Part print with two shaded views. Sizes in mm from the minimum x, y, z corner. Give positions to 0.01 mm unless a question says otherwise; leave off trailing zeros. Order: outer loops, then holes, each group sorted by start corner. A loop starts at its lowest first (then second) coordinate and runs counter-clockwise, first axis right, second up. Notation, with made-up numbers: M 5.5,-13 L 25.5,-13 A29 ccw 25.5,21 Z; hole C 31,-23.75 d7. An arc over 180 degrees is marked long. Return JSON: item names as keys, results as strings. Group by question number.
1. Pin check, flat tips, straight feed: pin 1 (1 mm diameter, centred on y = 0.5, z = 2.5, fed in from -X); pin 2 (1.2 mm diameter, centred on y = 29.5, z = 2, fed in from +X); pin 3 (2 mm diameter, centred on x = 19.5, z = 1, fed in from -Y); pin 4 (3.5 mm diameter, centred on x = 5, y = 8.5, fed in from +Z). Stop position of each tip, or through.
2. Slice it at D-D on y = 44. List the corners of the cut face in (x, z).
3. Slice it at B-B on z = 3.35. Give the number of separate pieces and of enclosed holes in the cut face, then the cut area to 3 significant figures.
4. Slice it at A-A on y = 8.5. List the corners of the cut face in (x, z).
5. Wall check: probe 1 along Y at (x, z) = (131, 1.8); probe 2 along X at (y, z) = (67, 1.4); probe 3 along Y at (x, z) = (153, 2.15). Give the ranges that are in metal, low to high. Write a range as [from, to].
6. Slice it at C-C on x = 5. List the corners of the cut face in (y, z), then the cut area to 3 significant figures.
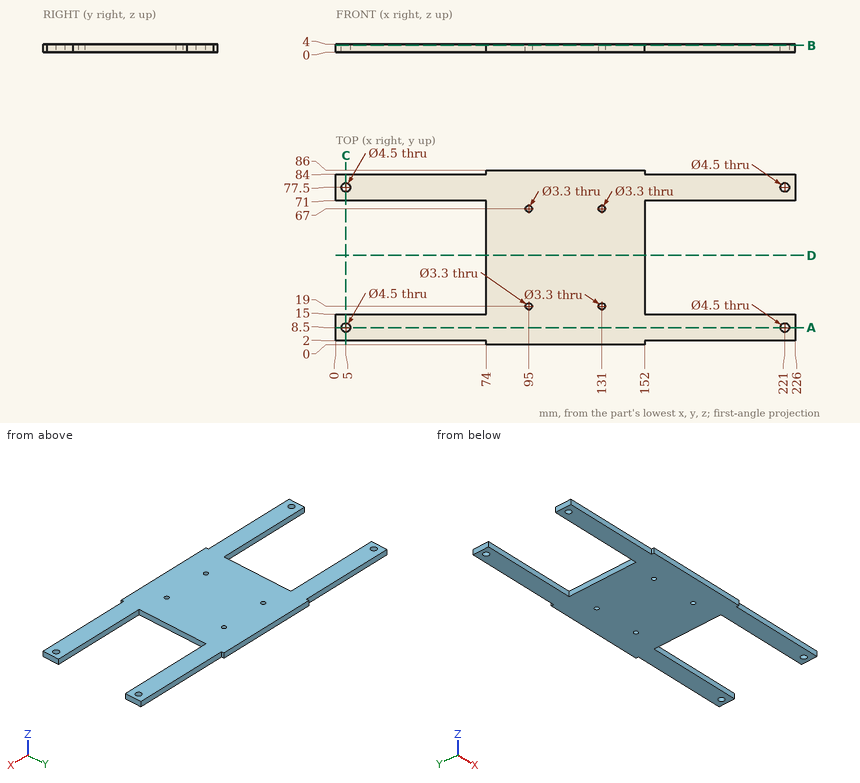
Result:
{
 "1": {"pin 1": "stops at x = 74", "pin 2": "stops at x = 152", "pin 3": "stops at y = 2", "pin 4": "passes through"},
 "2": {"outline": "M 74,0 L 152,0 L 152,4 L 74,4 Z"},
 "3": {"separate pieces": "1", "enclosed holes": "8", "area": "10,500 mm2"},
 "4": {"outline": "M 0,0 L 2.75,0 L 2.75,4 L 0,4 Z; M 7.25,0 L 218.75,0 L 218.75,4 L 7.25,4 Z; M 223.25,0 L 226,0 L 226,4 L 223.25,4 Z"},
 "5": {"probe 1": "y = [0, 17.35], [20.65, 65.35], [68.65, 86]", "probe 2": "x = [74, 93.35], [96.65, 129.35], [132.65, 152]", "probe 3": "y = [2, 15], [71, 84]"},
 "6": {"outline": "M 2,0 L 6.25,0 L 6.25,4 L 2,4 Z; M 10.75,0 L 15,0 L 15,4 L 10.75,4 Z; M 71,0 L 75.25,0 L 75.25,4 L 71,4 Z; M 79.75,0 L 84,0 L 84,4 L 79.75,4 Z", "area": "68.0 mm2"}
}
